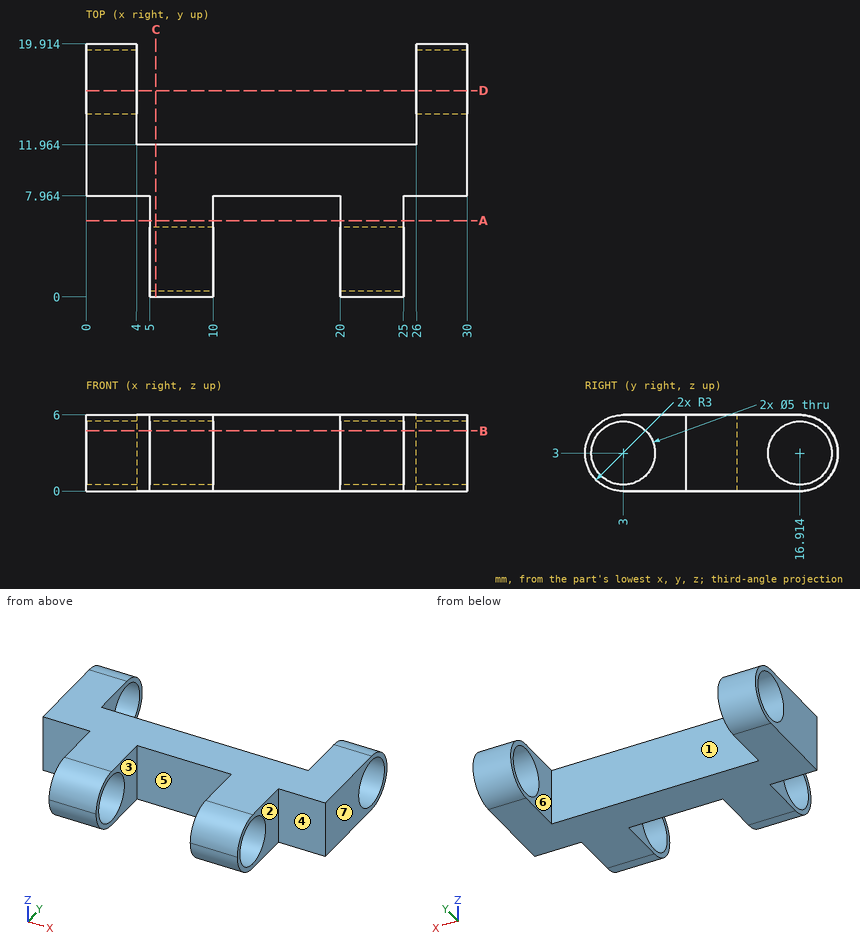
Can you work these out from the drawing? Everything is in mm from the part's minimum corner. A direction names the side the tool comes from. Round coordinates to 2 decimals unless told otherwise and drop trailing zeros. Order: outer loops, then holes, each group sorted by start corner. A loop starts at its lowest first (then second) coordinate and runs counter-clockwise, first axis right, second up.
(1) We'd pull the mould along X, two halves only. Please class the marked faces 4, 5, 6 and 7: +X half, -X half, draft (parallel to the pull), parting line (faces both ways), or undercut.
Results are:
face 4: draft
face 5: undercut
face 6: undercut
face 7: +X half
(2) If we section it at C-C (x = 5.5): Please give me the cut outline in (y, z).
Results are:
outline: (0, 3) arc R3 ccw to (3, 0) - (11.96, 0) - (11.96, 6) - (3, 6) arc R3 ccw to start; hole circle Ø5 at (3, 3)
(3) If I drill on L1, parallel to Z at x = 22.6, y = 3; L2, parallel to X at y = 5.75, z = 4.75; L3, parallel to X at y = 15.25, z = 0.75, over which ranges is the centre line in solid material (lowest first)?
Results are:
L1: z = 0 to 0.5, 5.5 to 6
L2: x = 5 to 10, 20 to 25
L3: x = 0 to 4, 26 to 30
(4) I'm going to push flat-ended pins straight in: pin 1 (1.5 mm diameter, centred on x = 3.5, z = 3.5, fed in from -Y); pin 2 (3 mm diameter, centred on y = 3.5, z = 4, fed in from +X); pin 3 (3 mm diameter, centred on y = 4, z = 3.5, fed in from -X); pin 4 (3 mm diameter, centred on y = 15.5, z = 3, fed in from +X). Where does each tip first touch, or does it pass through?
Results are:
pin 1: stops at y = 7.96
pin 2: stops at x = 25
pin 3: stops at x = 5
pin 4: stops at x = 30
(5) If we section it at D-D (y = 16.25): Please give me the cut outline in (x, z).
Results are:
outline: (0, 0) - (4, 0) - (4, 0.59) - (0, 0.59) - close; (0, 5.41) - (4, 5.41) - (4, 6) - (0, 6) - close; (26, 0) - (30, 0) - (30, 0.59) - (26, 0.59) - close; (26, 5.41) - (30, 5.41) - (30, 6) - (26, 6) - close
(6) If we section it at B-B (z = 4.75): Count the separate pieces of the cut face and the enclosed holes in it, plus the area to 3 significant figures.
Results are:
separate pieces: 5
enclosed holes: 0
area: 189 mm2
(7) On a 3-axis mill with a long thin cutter (end or side, diameter ignored), from which of +Z, -Z, +X, -X, +Y, -Y can I reach the whole of each face in a straight line? I mean the marked faces 1, 2 and 3. Say none if no direction works.
Results are:
face 1: +Z, -Z, +Y
face 2: +Z, -Z, +X, -Y
face 3: +Z, -Z, -Y
(8) If we section it at A-A (y = 6): Please give me the cut outline in (x, z), plus the area to 3 significant figures.
Results are:
outline: (5, 0) - (10, 0) - (10, 6) - (5, 6) - close; (20, 0) - (25, 0) - (25, 6) - (20, 6) - close
area: 60.0 mm2
